from build123d import *

# Parameters (mm, degrees)
BOX_W       = 76.2
BOX_H       = 1590.55
BOX_DEPTH   = 76.2
THICKNESS_T = -6.35


with BuildPart() as part:
    # Box → Box (new body)
    with BuildSketch(Plane.XY):
        with Locations((38.1, 795.275)):
            Rectangle(BOX_W, BOX_H)
    extrude(amount=BOX_DEPTH)

    # Thickness
    thickness_openings = [part.faces().sort_by_distance(p)[0] for p in [
        (38.1, 0, 38.1),
        (38.1, 1590.55, 38.1),
    ]]
    offset(amount=THICKNESS_T, openings=thickness_openings)


solid = part.part
The listing builds one solid part. Answer for the finished solid, in the listing's coordinates (mm). A direction names the side the tool comes from. Coordinates: 2 decimals unless noted, no trailing zeros. Loops run counter-clockwise (first coordinate to the right, second up) from the corner with the lowest first, then second, coordinate; pieces in that order, holes last. Notation, with made-up numbers: M -39,69 L 5,69 A28 ccw 5,102 Z; hole C -24.5,-31.5 d8. An arc over 180 degrees is marked long. Answer in a Markdown table with one row per item.
1) Find the intervals of material crossed by probe 1 along X at (y, z) = (621, 58), in increasing order.
Answers below:
| item | result |
|---|---|
| probe 1 | 0 to 6.35, 69.85 to 76.2 |
2) Find section A-A (z = 20.5). Determine the outline of the cut face in (x, y), then the cut area to 3 significant figures.
Answers below:
| item | result |
|---|---|
| outline | M 0,0 L 6.35,0 L 6.35,1590.55 L 0,1590.55 Z; M 69.85,0 L 76.2,0 L 76.2,1590.55 L 69.85,1590.55 Z |
| area | 20,200 mm^2 |
3) Determine the mould class of faces 3 (the flat face through (71, 0, 38)), 4 (the flat face through (6.35, 784, 38)), 5 (the flat face through (76.2, 784, 38)), 6 (the flat face through (0, 784, 38)) for opening direction X: released by +X, released by -X, zero draft, split by the parting line, or undercut.
Answers below:
| item | result |
|---|---|
| face 3 | zero draft |
| face 4 | undercut |
| face 5 | released by +X |
| face 6 | released by -X |
4) Find section B-B (y = 675.5). Determine the outline of the cut face in (x, z), then the cut area to 3 significant figures.
Answers below:
| item | result |
|---|---|
| outline | M 0,0 L 76.2,0 L 76.2,76.2 L 0,76.2 Z; hole M 6.35,6.35 L 69.85,6.35 L 69.85,69.85 L 6.35,69.85 Z |
| area | 1,770 mm^2 |
5) Which of the six approach directions +Z, -Z, +X, -X, +Y, -Y give full straight-line access (tool end or side, diameter ignored) to faces 1 (the flat face through (38, 806, 0)), 2 (the flat face through (38, 806, 6.35))?
Answers below:
| item | result |
|---|---|
| face 1 | -Z, +X, -X, +Y, -Y |
| face 2 | +Y, -Y |
